Answer from the drawing. Dimensions are ordinates in mm from the lowest x, y and z of the part. A direction names the side the tool comes from. Coordinates: 2 decimals unless noted, no trailing zeros. Loops run counter-clockwise (first coordinate to the right, second up) from the corner with the lowest first, then second, coordinate; pieces in that order, holes last.
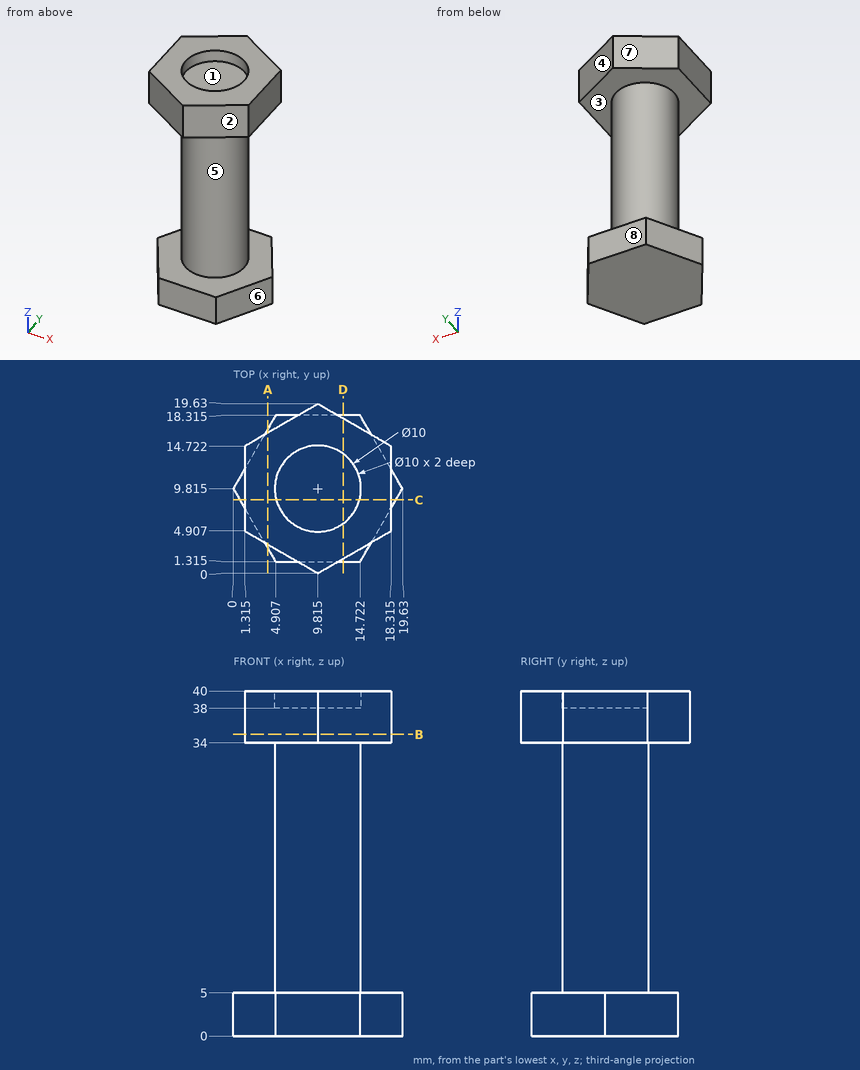
Item 1: Determine the mould class of the marked faces 1, 2 and 3 for opening direction Z: released by +Z, released by -Z, zero draft, split by the parting line, or undercut.
Numbers:
face 1: released by +Z
face 2: zero draft
face 3: undercut
Item 2: Find the intervals of material crossed by line 1 along Z through (x, y) = (17.75, 10); line 2 along X through (y, z) = (13.25, 36) (1 decimal); line 3 along Z through (x, y) = (2, 6), in increasing order.
Numbers:
line 1: z = 0 to 5, 34 to 40
line 2: x = 1.3 to 18.3
line 3: z = 34 to 40
Item 3: Given pin 1 (5.5 mm diameter, centred on x = 11.5, z = 3, fed in from +Y) (1 decimal); pin 2 (6.5 mm diameter, centred on y = 7.5, z = 37, fed in from +X) (1 decimal); pin 3 (3 mm diameter, centred on y = 10, z = 36.5, fed in from -X) (1 decimal), each flat-ended and moving along its own axis, determine where each tip first touches the part or whether it passes through.
Numbers:
pin 1: stops at y = 18.3
pin 2: stops at x = 18.3
pin 3: stops at x = 1.3
Item 4: Which of the six approach directions +Z, -Z, +X, -X, +Y, -Y give full straight-line access (tool end or side, diameter ignored) to the marked faces 4, 5, 6, 7 and 8?
Numbers:
face 4: +Z, +X, +Y
face 5: none
face 6: -Z, +X, -Y
face 7: +Z, -X, +Y
face 8: -Z, +X, -X, +Y
Item 5: A cutting plane is placed at C-C on y = 8.5. Determine the outline of the cut face in (x, z) (1 decimal), then the cut area to 3 significant figures.
Numbers:
outline: (0.8, 0) - (18.9, 0) - (18.9, 5) - (14.6, 5) - (14.6, 34) - (18.3, 34) - (18.3, 40) - (14.6, 40) - (14.6, 38) - (5, 38) - (5, 40) - (1.3, 40) - (1.3, 34) - (5, 34) - (5, 5) - (0.8, 5) - close
area: 453 mm2
Item 6: A cutting plane is placed at A-A on x = 4. Determine the outline of the cut face in (y, z), then the cut area to 3 significant figures.
Numbers:
outline: (2.89, 0) - (16.74, 0) - (16.74, 5) - (2.89, 5) - close; (3.36, 34) - (16.27, 34) - (16.27, 40) - (3.36, 40) - close
area: 147 mm2
Item 7: A cutting plane is placed at D-D on x = 12.75. Determine the outline of the cut face in (y, z) (1 decimal).
Numbers:
outline: (1.3, 0) - (18.3, 0) - (18.3, 5) - (13.9, 5) - (13.9, 34) - (17.9, 34) - (17.9, 40) - (13.9, 40) - (13.9, 38) - (5.8, 38) - (5.8, 40) - (1.7, 40) - (1.7, 34) - (5.8, 34) - (5.8, 5) - (1.3, 5) - close
Item 8: A cutting plane is placed at B-B on z = 35. Determine the outline of the cut face in (x, y) (1 decimal).
Numbers:
outline: (1.3, 4.9) - (9.8, 0) - (18.3, 4.9) - (18.3, 14.7) - (9.8, 19.6) - (1.3, 14.7) - close
